Read the model definition and answer for the solid it produces. Units are mm, in the model's axes. A direction names the side the tool comes from. Coordinates: 2 decimals unless noted, no trailing zeros. Order: outer loops, then holes, each group sorted by start corner. A loop starts at its lowest first (then second) coordinate and runs counter-clockwise, first axis right, second up.
from build123d import *

# Parameters (mm, degrees)
SKETCH1_R           = 2.2
SKETCH1_R_2         = 1.25
BOSS_EXTRUDE1_DEPTH = 12
SKETCH2_R           = 3
SKETCH2_R_2         = 0.675
BOSS_EXTRUDE2_DEPTH = 7
CUT_EXTRUDE1_DEPTH  = 8.9


with BuildPart() as part:
    # Sketch1 → Boss-Extrude1 (new body)
    with BuildSketch(Plane.XY):
        Circle(SKETCH1_R)
        Circle(SKETCH1_R_2, mode=Mode.SUBTRACT)
    extrude(amount=BOSS_EXTRUDE1_DEPTH)

    # Sketch2 → Boss-Extrude2 (add)
    with BuildSketch(Plane.XY.offset(12)):
        Circle(SKETCH2_R)
        Circle(SKETCH2_R_2, mode=Mode.SUBTRACT)
    extrude(amount=BOSS_EXTRUDE2_DEPTH)

    # Sketch3 → Cut-Revolve1 (revolve, cut)
    with BuildSketch(Plane(origin=(0, 0, 0), x_dir=(1, 0, 0), z_dir=(0, 1, 0))):
        Polygon((2.2, -12), (3, -13), (4.276308893, -12.361058563), (3.46784885, -11.152134436), align=None)
        Polygon((2.375, -19), (3, -16), (5.751760011, -17.171813113), (4.254862661, -20.939605223), align=None)
    revolve(axis=Axis((0, 0, 0), (0, 0, 1)), mode=Mode.SUBTRACT)

    # Sketch4 → Cut-Extrude1 (cut)
    with BuildSketch(Plane.XY.offset(19)):
        Polygon((0, 3.340763125), (-0.25, 3.340763125), (-0.25, 0.464842209), (0.25, 0.464842209), (0.25, 3.340763125), align=None)
        Polygon((3.340763125, 0), (3.340763125, 0.25), (0.464842209, 0.25), (0.464842209, -0.25), (3.340763125, -0.25), align=None)
        Polygon((0, -3.340763125), (0.25, -3.340763125), (0.25, -0.464842209), (-0.25, -0.464842209), (-0.25, -3.340763125), align=None)
        Polygon((-3.340763125, 0), (-3.340763125, -0.25), (-0.464842209, -0.25), (-0.464842209, 0.25), (-3.340763125, 0.25), align=None)
    extrude(amount=-CUT_EXTRUDE1_DEPTH, mode=Mode.SUBTRACT)


solid = part.part
Q1. The part is cut by section D-D, the plane z = 1.5. Determine the outline of the cut face in (x, y).
Q2. Which of the six approach directions +Z, -Z, +X, -X, +Y, -Y give full straight-line access (tool end or side, diameter ignored) to faces 4 (the conical face through (-1.8, -1.76, 12.4)), 5 (the conical face through (-1.9, -1.9, 17.5)), 6 (the flat face through (-0.25, -2, 15)), 7 (the flat face through (2, -0.25, 15)), 8 (the cylindrical face through (2.1, 0.66, 5.92))?
Q3. Each of these flat-tipped pins is pushed along its axis until it touches: P1, Ø1.2, axis at y = 2.5, z = 12.5, coming from the -X side; P2, Ø1.9, axis at x = -1.5, z = 15.5, coming from the +Y side; P3, Ø0.7, axis at x = -2.5, z = 13, coming from the -Y side. Where does it stop, or does it pass through?
Q4. Straight lines are drawn through the part: L1, parallel to Y at x = 0, z = 5; L2, parallel to Y at x = -2.15, z = 17.25. For each, find the intervals that lie inside material, in ascending order.
Q5. Determine the mould class of faces 1 (the flat face through (-0.6, -0.6, 12)), 2 (the conical face through (-1.76, 1.8, 12.4)), 3 (the cylindrical face through (-2.14, -2.1, 14.48)) for opening direction Y: +Y half, -Y half, draft (parallel to the pull), parting line (faces both ways), or undercut.
Q6. The part is cut by section C-C, the plane z = 16.5. Determine the outline of the cut face in (x, y) (3 decimals).
Q7. The part is cut by section A-A, the plane y = 0. Determine the outline of the cut face in (x, z).
Computed values:
1. outline: circle Ø4.4 at (0, 0); hole circle Ø2.5 at (0, 0)
2. face 4: -Z, -X, -Y
2. face 5: +Z, -X, -Y
2. face 6: +Z, +Y, -Y
2. face 7: +Z, +X, -X
2. face 8: -Z
3. P1: stops at x = -2.08
3. P2: stops at y = 2.95
3. P3: stops at y = -2.09
4. L1: y = -2.2 to -1.25, 1.25 to 2.2
4. L2: y = -1.7 to -0.25, 0.25 to 1.7
5. face 1: undercut
5. face 2: +Y half
5. face 3: -Y half
6. outline: (-2.885, -0.25) arc R2.896 ccw to (-0.25, -2.885) - (-0.25, -0.627) arc R0.675 cw to (-0.627, -0.25) - close; (-2.885, 0.25) - (-0.627, 0.25) arc R0.675 cw to (-0.25, 0.627) - (-0.25, 2.885) arc R2.896 ccw to start; (0.25, -2.885) arc R2.896 ccw to (2.885, -0.25) - (0.627, -0.25) arc R0.675 cw to (0.25, -0.627) - close; (0.25, 0.627) arc R0.675 cw to (0.627, 0.25) - (2.885, 0.25) arc R2.896 ccw to (0.25, 2.885) - close
7. outline: (-2.2, 0) - (-1.25, 0) - (-1.25, 10.1) - (-2.2, 10.1) - close; (1.25, 0) - (2.2, 0) - (2.2, 10.1) - (1.25, 10.1) - close
